Drawing for the job (mm, zero at the part's lowest x, y, z). A direction names the side the tool comes from. Give positions to 0.01 mm unless a question says otherwise; leave off trailing zeros. Order: outer loops, then holes, each group sorted by start corner. A loop starts at its lowest first (then second) coordinate and runs counter-clockwise, first axis right, second up. Notation, with made-up numbers: (80.25, 18.5) - (118.25, 18.5) arc R21 cw to (118.25, 28.5) - close; hole circle Ø10 at (81, 34.5). An arc over 180 degrees is marked (long way). One line per item, written item: value.
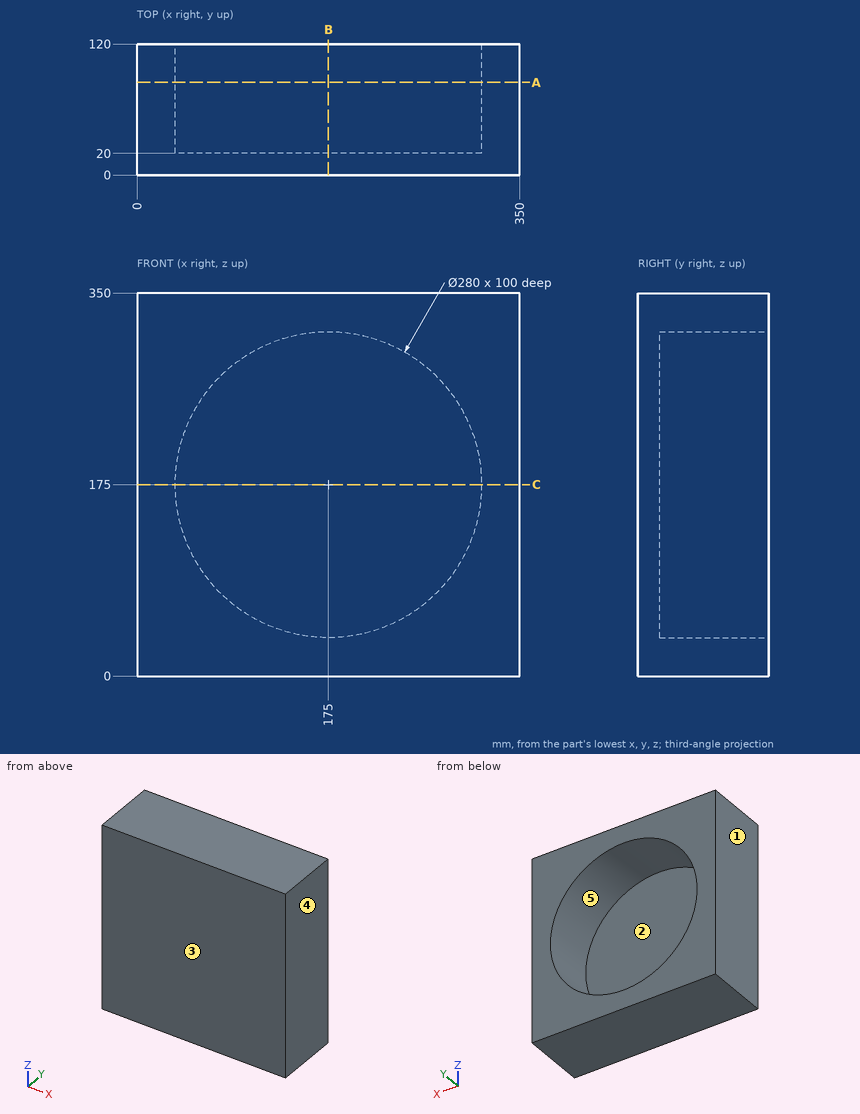
(1) 3-axis set-ups, long thin cutter, end or side, ignore diameter. For the marked faces 1 and 2: which of +Z, -Z, +X, -X, +Y, -Y reach the whole face in a straight line?
Completed:
face 1: +Z, -Z, -X, +Y, -Y
face 2: +Y
(2) Slice it at C-C, the plane z = 175. Give the cut face in (x, y), and give its area (3 significant figures).
Completed:
outline: (0, 0) - (350, 0) - (350, 120) - (315, 120) - (315, 20) - (35, 20) - (35, 120) - (0, 120) - close
area: 14,000 mm²
(3) Pull direction X, two halves, no side cores. Call the marked faces 3, 4 and 5: +X half, -X half, draft (parallel to the pull), parting line (faces both ways), or undercut.
Completed:
face 3: draft
face 4: +X half
face 5: undercut
(4) Slice it at B-B, the plane x = 175. Give the cut face in (y, z), and give its area (3 significant figures).
Completed:
outline: (0, 0) - (120, 0) - (120, 35) - (20, 35) - (20, 315) - (120, 315) - (120, 350) - (0, 350) - close
area: 14,000 mm²
(5) Slice it at A-A, the plane y = 85. Give the cut face in (x, z).
Completed:
outline: (0, 0) - (350, 0) - (350, 350) - (0, 350) - close; hole circle Ø280 at (175, 175)
(6) Drill centre lines: line 1 (X direction, y = 61.5, z = 175); line 2 (Z direction, x = 88.5, y = 72). Where is each one in solid material? Low to high.
Completed:
line 1: 0 to 35, 315 to 350
line 2: 0 to 64.92, 285.08 to 350
